Verification items for the finished model (mm, model axes). A direction names the side the tool comes from. Round coordinates to 2 decimals unless told otherwise and drop trailing zeros. Order: outer loops, then holes, each group sorted by start corner. A loop starts at its lowest first (then second) coordinate and runs counter-clockwise, first axis right, second up. Notation, with made-up numbers: M 70.25,10.5 L 114.25,10.5 A15 cw 114.25,17.5 Z; hole C -33,65 d10. An arc over 180 degrees is marked long. Use one line per item in the form item = value. Start each with the question number.
Item 1: Cross-section at D-D on y = -34.5. Enter the section's corners in (x, z), then the cut area to 3 significant figures.
Item 2: Release check for a two-part mould opening along X. For faces 1 (the flat face through (6, 1, 0)), 2 (the flat face through (3.892, 34.446, 0.76)), 3 (the flat face through (-31, -1, 6)), 4 (the flat face through (6, 1, 1.5)) record: +X half, -X half, draft (parallel to the pull), parting line (faces both ways), or undercut.
Item 3: Cross-section at C-C on y = 20.5. Enter the section's corners in (x, z), then the cut area to 3 significant figures.
Item 4: Cross-section at A-A on z = 4. Enter the section's corners in (x, y).
Item 5: Thickness scan on probe 1 along X at (y, z) = (-32.5, 4.5); probe 2 along Y at (x, z) = (7, 1.2); probe 3 along Y at (x, z) = (-15, 0.8). Record the ranges inside material, lowest first. Write a range as [from, to].
Item 6: Tool access check on faces 5 (the flat face through (-29.5, 1, 7)), 6 (the cylindrical face through (-6.75, 24.91, 0.76)), 7 (the flat face through (-2, -46, 1)). Record the directions out of +Z, -Z, +X, -X, +Y, -Y that give a thin tool (end or side, any length) a straight path to the whole face; none if there is none.
Item 7: Cross-section at B-B on x = 7. Enter the section's corners in (y, z), then the cut area to 3 significant figures.
Item 8: Go/stop test with flat-tipped pins: pin 1 Ø1.5 at (y, z) = (23, 9) entering from +X; pin 2 Ø1.6 at (x, y) = (30.5, 13.5) entering from +Z; pin 3 Ø2.5 at (x, y) = (7, 26) entering from -Z; pin 4 Ø10 at (x, y) = (4, -7) entering from +Z. Record where each tip stops, or that it passes through.
Autodesk Inventor part; units mm, degrees
ref_plane "YZ Plane" through (0, 0, 0) normal (1, 0, 0) x (0, 1, 0)
ref_plane "XZ Plane" through (0, 0, 0) normal (0, 1, 0) x (-1, 0, 0)
ref_plane "XY Plane" through (0, 0, 0) normal (0, 0, 1) x (1, 0, 0)
sketch "スケッチ1" plane through (0, 0, 0) normal (0, 0, 1) x (1, 0, 0)
  line L0 (-31, 46) -> (31, 46)
  line L1 (31, 46) -> (31, -46)
  line L2 (31, -46) -> (-31, -46)
  line L3 (-31, -46) -> (-31, 46)
  point P0 (0, 0)
  dimension "d0" = 92
  dimension "d1" = 46
  dimension "d2" = 62
  dimension "d3" = 31
extrude "押し出し1" add sketch "スケッチ1" along normal blind 1.5
sketch "スケッチ3" plane through (0, 0, 0) normal (0, 0, -1) x (-1, 0, 0)
  circle A0 centre (-7, 26) radius 1.5
  circle A1 centre (15, 26) radius 1.5
  circle A2 centre (-7, -12) radius 1.5
  circle A3 centre (15, -12) radius 1.5
  line L0 (31, 46) -> (-31, 46)
  line L1 (31, -46) -> (31, 46)
  point P0 (0, 0)
  dimension "d10" = 3
  dimension "d11" = 22
  dimension "d12" = 22
  dimension "d15" = 38
  dimension "d16" = 38
  dimension "d35" = 20
  dimension "d36" = 20
  dimension "d44" = 16
  dimension "d45" = 16
hole "穴1" at (-15, -12, 0) at (-15, 26, 0) at (7, 26, 0) at (7, -12, 0) direction (0, 0, 1) diameter 3 end through all
sketch "スケッチ4" plane through (0, 0, 1.5) normal (0, 0, 1) x (1, 0, 0)
  line L0 (-31, -46) -> (-31, 46)
  line L1 (31, -46) -> (-31, -46)
  line L2 (-31, 46) -> (-29.5, 46)
  line L3 (-29.5, 46) -> (-29.5, -46)
  line L4 (-29.5, -46) -> (-31, -46)
  line L5 (-31, -46) -> (-31, 46)
  line L6 (31, 46) -> (29.5, 46)
  line L7 (29.5, 46) -> (29.5, -46)
  line L8 (29.5, -46) -> (31, -46)
  line L9 (31, -46) -> (31, 46)
  point P0 (0, 0)
  dimension "d37" = 59
  dimension "d39" = 1.5
extrude "押し出し3" add sketch "スケッチ4" along normal blind 11
sketch "スケッチ6" plane through (31, -46, 0) normal (1, 0, 0) x (0, 0, -1)
  line L0 (0, 0) -> (-12.5, 0)
  line L1 (-12.5, 92) -> (-6.25, 92)
  line L2 (-6.25, 92) -> (-6.25, 0)
  line L3 (-6.25, 0) -> (-12.5, 0)
  line L4 (-12.5, 0) -> (-12.5, 92)
  point P0 (0, 46)
extrude "押し出し5" cut sketch "スケッチ6" against normal blind 1.5
sketch "スケッチ7" plane through (0, 0, 1.5) normal (0, 0, 1) x (1, 0, 0)
  line L0 (-29.5, 46) -> (-29.5, -46)
  line L1 (29.5, -46) -> (29.5, 46)
  line L2 (4.5, 13.4115) -> (4.5, 1.4115)
  line L3 (-18.5, 1.4115) -> (-18.5, 13.4115)
  line L4 (-19, 36.9115) -> (8, 36.9115)
  line L5 (-0.3333, 31.9115) -> (-16, 31.9115)
  line L6 (-16, -18.9115) -> (4, -18.9115)
  line L7 (16, -36.9115) -> (-24, -36.9115)
  line L8 (-24, -36.9115) -> (-16, -18.9115)
  line L9 (16, -36.9115) -> (4, -18.9115)
  line L10 (31, 18.1628) -> (29.5, 17.5573)
  line L11 (-19, 36.9115) -> (-16, 31.9115)
  line L12 (8, 36.9115) -> (-0.3333, 31.9115)
  arc A0 (-18.5, 1.4115) -> (4.5, 1.4115) centre (-7, 1.4115) ccw
  arc A1 (4.5, 13.4115) -> (-18.5, 13.4115) centre (-7, 13.4115) ccw
  line L13 (31, 46) -> (31, -46)
  line L14 (12, -10.9115) -> (23.5, -28.1615)
  line L15 (23.5, -28.1615) -> (23.5, 26.8385)
  line L16 (23.5, 26.8385) -> (12, 24.0885)
  line L17 (12, -10.9115) -> (12, 24.0885)
  line L18 (29.5, -46) -> (29.5, 46)
  line L19 (-29.5, 46) -> (29.5, 46)
  line L20 (29.5, -46) -> (-29.5, -46)
  point P0 (0, 0)
  point P1 (-31, 0)
  point P2 (31, 43.9415)
  point P3 (31, -43.9415)
  point P4 (29.5, -43.9415)
  point P5 (29.5, 43.9415)
  dimension "d62" = 12
  dimension "d63" = 11.5
  dimension "d64" = 11.5
  dimension "d65" = 23
  dimension "d70" = 5
  dimension "d72" = 18
  dimension "d73" = 27
  dimension "d78" = 13.5
  dimension "d79" = 10.5
  dimension "d80" = 11
  dimension "d89" = 40
  dimension "d92" = 20
  dimension "d114" = 35
  dimension "d115" = 55
  dimension "d118" = 11.5
  dimension "d119" = 6
  dimension "d125" = 9.0885
  dimension "d126" = 9.0885
  dimension "d127" = 47.4115
  dimension "d128" = 21.9115
  dimension "d129" = 38
  dimension "d130" = 27
  dimension "d131" = 15
  dimension "d132" = 38
extrude "押し出し6" cut sketch "スケッチ7" against normal blind 1.5 contours L2 A0 L3 A1 | L4 L12 L5 L11 | L6 L9 L7 L8 | L17 L16 L15 L14
properties part number "16" material "アルミニウム 6061"
Output values:
q1.outline = M -31,0 L -22.93,0 L -22.93,1.5 L -29.5,1.5 L -29.5,12.5 L -31,12.5 Z; M 14.39,0 L 31,0 L 31,6.25 L 29.5,6.25 L 29.5,1.5 L 14.39,1.5 Z
q1.area = 60.6 mm2
q2.face_1 = draft
q2.face_2 = undercut
q2.face_3 = -X half
q2.face_4 = undercut
q3.outline = M -31,0 L -16.06,0 L -16.06,1.5 L -29.5,1.5 L -29.5,12.5 L -31,12.5 Z; M 2.06,0 L 12,0 L 12,1.5 L 2.06,1.5 Z; M 23.5,0 L 31,0 L 31,6.25 L 29.5,6.25 L 29.5,1.5 L 23.5,1.5 Z
q3.area = 72.2 mm2
q4.outline = M -31,-46 L -29.5,-46 L -29.5,46 L -31,46 Z; M 29.5,-46 L 31,-46 L 31,46 L 29.5,46 Z
q5.probe_1 = [-31, -29.5], [29.5, 31]
q5.probe_2 = [-46, -36.91], [-23.41, -13.5], [-10.5, 24.5], [27.5, 36.31], [36.91, 46]
q5.probe_3 = [-46, -36.91], [-18.91, -13.5], [-10.5, -6.85], [21.67, 24.5], [27.5, 31.91], [36.91, 46]
q6.face_5 = +Z, +Y, -Y
q6.face_6 = +Z, -Z
q6.face_7 = +Z, -Z, +X, -X, -Y
q7.outline = M -46,0 L -36.91,0 L -36.91,1.5 L -46,1.5 Z; M -23.41,0 L -13.5,0 L -13.5,1.5 L -23.41,1.5 Z; M -10.5,0 L 24.5,0 L 24.5,1.5 L -10.5,1.5 Z; M 27.5,0 L 36.31,0 L 36.31,1.5 L 27.5,1.5 Z; M 36.91,0 L 46,0 L 46,1.5 L 36.91,1.5 Z
q7.area = 108 mm2
q8.pin_1 = -29.5
q8.pin_2 = 6.25
q8.pin_3 = through
q8.pin_4 = 1.5
